```python
from build123d import *

# Parameters (mm, degrees)
SKETCH2_R           = 30
BOSS_EXTRUDE1_DEPTH = 30
SKETCH3_W           = 13.5
SKETCH3_H           = 15
CUT_EXTRUDE1_DEPTH  = 31
SKETCH4_W           = 33
SKETCH4_H           = 13.5
CUT_EXTRUDE2_DEPTH  = 10.5
SKETCH5_W           = 25
SKETCH5_H           = 13.5
CUT_EXTRUDE3_DEPTH  = 20.5
FILLET1_R           = 0.5
BOSS_EXTRUDE2_DEPTH = 2.5
SKETCH9_R           = 2.75
CUT_EXTRUDE4_DEPTH  = 3.5
SKETCH10_R          = 1.5
CUT_EXTRUDE5_DEPTH  = 5
FILLET2_R           = 2


with BuildPart() as part:
    # Sketch2 → Boss-Extrude1 (new body)
    with BuildSketch(Plane(origin=(0, 0, 0), x_dir=(1, 0, 0), z_dir=(0, 1, 0))):
        Circle(SKETCH2_R)
    extrude(amount=BOSS_EXTRUDE1_DEPTH)

    # Sketch3 → Cut-Extrude1 (cut, through all)
    with BuildSketch(Plane(origin=(0, 0, 0), x_dir=(0, 0, -1), z_dir=(1, 0, 0))):
        with Locations((0, 7.5)):
            Rectangle(SKETCH3_W, SKETCH3_H)
    extrude(amount=CUT_EXTRUDE1_DEPTH, mode=Mode.SUBTRACT)

    # Sketch4 → Cut-Extrude2 (cut)
    with BuildSketch(Plane(origin=(0, 30, 0), x_dir=(1, 0, 0), z_dir=(0, 1, 0))):
        with Locations((-5.5, 0)):
            Rectangle(SKETCH4_W, SKETCH4_H)
    extrude(amount=-CUT_EXTRUDE2_DEPTH, mode=Mode.SUBTRACT)

    # Sketch5 → Cut-Extrude3 (cut, through all)
    with BuildSketch(Plane(origin=(0, 19.5, 0), x_dir=(1, 0, 0), z_dir=(0, 1, 0))):
        with Locations((-5.5, 0)):
            Rectangle(SKETCH5_W, SKETCH5_H)
    extrude(amount=-CUT_EXTRUDE3_DEPTH, mode=Mode.SUBTRACT)

    # Sketch7 → Revolve1 (revolve)
    with BuildSketch(Plane.XY):
        with BuildLine():
            Line((30, 30), (28, 30))
            Line((28, 30), (28, 32))
            ThreePointArc((28, 32), (29, 33), (30, 32))
            Line((30, 32), (30, 30))
        make_face()
    revolve(axis=Axis((0, 34.959815409, 0), (0, -1, 0)))

    # Fillet1
    fillet1_edges = [part.edges().sort_by_distance(p)[0] for p in [
        (-28, 30, 0),
    ]]
    fillet(fillet1_edges, radius=FILLET1_R)

    # Sketch8 → Boss-Extrude2 (add)
    with BuildSketch(Plane(origin=(0, 0, 0), x_dir=(1, 0, 0), z_dir=(0, 1, 0))):
        with BuildLine():
            ThreePointArc((24.452034569, -17.380966757), (21.213203436, -21.213203436), (17.380966757, -24.452034569))
            Line((17.380966757, -24.452034569), (24.452034569, -31.523102381))
            ThreePointArc((24.452034569, -31.523102381), (31.523102381, -31.523102381), (31.523102381, -24.452034569))
            Line((31.523102381, -24.452034569), (24.452034569, -17.380966757))
        make_face()
        with BuildLine():
            ThreePointArc((-17.380966757, -24.452034569), (-21.213203436, -21.213203436), (-24.452034569, -17.380966757))
            Line((-24.452034569, -17.380966757), (-31.523102381, -24.452034569))
            ThreePointArc((-31.523102381, -24.452034569), (-31.523102381, -31.523102381), (-24.452034569, -31.523102381))
            Line((-24.452034569, -31.523102381), (-17.380966757, -24.452034569))
        make_face()
        with BuildLine():
            ThreePointArc((17.380966757, 24.452034569), (21.213203436, 21.213203436), (24.452034569, 17.380966757))
            Line((24.452034569, 17.380966757), (31.523102381, 24.452034569))
            ThreePointArc((31.523102381, 24.452034569), (31.523102381, 31.523102381), (24.452034569, 31.523102381))
            Line((24.452034569, 31.523102381), (17.380966757, 24.452034569))
        make_face()
        with BuildLine():
            ThreePointArc((-24.452034569, 17.380966757), (-21.213203436, 21.213203436), (-17.380966757, 24.452034569))
            Line((-17.380966757, 24.452034569), (-24.452034569, 31.523102381))
            ThreePointArc((-24.452034569, 31.523102381), (-31.523102381, 31.523102381), (-31.523102381, 24.452034569))
            Line((-31.523102381, 24.452034569), (-24.452034569, 17.380966757))
        make_face()
    extrude(amount=BOSS_EXTRUDE2_DEPTH)

    # Sketch9 → Cut-Extrude4 (cut, through all)
    with BuildSketch(Plane(origin=(0, 2.5, 0), x_dir=(1, 0, 0), z_dir=(0, 1, 0))):
        with Locations((-27.987568475, 27.987568475)):
            Circle(SKETCH9_R)
        with Locations((27.987568475, 27.987568475)):
            Circle(SKETCH9_R)
        with Locations((27.987568475, -27.987568475)):
            Circle(SKETCH9_R)
        with Locations((-27.987568475, -27.987568475)):
            Circle(SKETCH9_R)
    extrude(amount=-CUT_EXTRUDE4_DEPTH, mode=Mode.SUBTRACT)

    # Sketch10 → Cut-Extrude5 (cut)
    with BuildSketch(Plane(origin=(0, 19.5, 0), x_dir=(1, 0, 0), z_dir=(0, 1, 0))):
        with Locations((-20, 0)):
            Circle(SKETCH10_R)
        with Locations((9, 0)):
            Circle(SKETCH10_R)
    extrude(amount=-CUT_EXTRUDE5_DEPTH, mode=Mode.SUBTRACT)

    # Fillet2
    fillet2_edges = [part.edges().sort_by_distance(p)[0] for p in [
        (-21.213203436, 2.5, -21.213203436),
        (21.213203436, 2.5, 21.213203436),
        (-21.213203436, 2.5, 21.213203436),
        (21.213203436, 2.5, -21.213203436),
    ]]
    fillet(fillet2_edges, radius=FILLET2_R)


solid = part.part
```
Read the model definition and answer for the solid it produces. Units are mm, in the model's axes. A direction names the side the tool comes from. Give positions to 0.01 mm unless a question says otherwise; leave off trailing zeros. Loops run counter-clockwise (first coordinate to the right, second up) from the corner with the lowest first, then second, coordinate; pieces in that order, holes last.
Item 1: The part is cut by section B-B (y = 16.5). Write down the section's boundary in (x, z), and give its area (3 significant figures).
Item 2: The part is cut by section C-C (z = 0). Write down the section's boundary in (x, y).
Item 3: Each of these flat-tipped pins is pushed along its axis until it touches: pin 1 Ø10 at (x, y) = (-19, 25) entering from -Z; pin 2 Ø8 at (y, z) = (7.5, -24.5) entering from +X; pin 3 Ø4.5 at (x, z) = (-26.5, -25) entering from +Y; pin 4 Ø6 at (x, z) = (-22.5, 8.5) entering from -Y. Where does it stop, or does it pass through?
Item 4: For faces 4 (the flat face through (20.87, 1.22, 27.94)), 5 (the cylindrical face through (-21.5, 17.04, -0.07)), 6 (the flat face through (27.94, 1.22, -20.87)), 7 (the cylindrical face through (-30.014, 1.268, 26.129)), determine the directions among +Z, -Z, +X, -X, +Y, -Y from which every point of the face is accessible in a straight line to the end or side of a thin tool.
Item 5: The part is cut by section D-D (y = 23). Write down the section's boundary in (x, z).
Item 6: The mould has two halves that part along Z. Classify faces 1 (the flat face through (-26, 2.5, -24)), 2 (the flat face through (-20.87, 1.22, -27.94)), 3 (the flat face through (-18, 10, 0)): released by +Z, released by -Z, zero draft, split by the parting line, or undercut.
Item 7: The part is cut by section A-A (x = 0). Write down the section's boundary in (y, z), and give its area (3 significant figures).
Item 8: Find the intervals of material crossed by line 1 along Z through (x, y) = (0, 30.9); line 2 along Z through (x, y) = (27.5, 11.5); line 3 along X through (y, z) = (31, 5.5), in increasing order.
Taken from the geometry:
1. outline: circle Ø60 at (0, 0); hole circle Ø3 at (-20, 0); hole (-18, -6.75) - (7, -6.75) - (7, 6.75) - (-18, 6.75) - close; hole circle Ø3 at (9, 0)
1. area: 2,480 mm2
2. outline: (-30, 0) - (-18, 0) - (-18, 19.5) - (-18.5, 19.5) - (-18.5, 14.5) - (-21.5, 14.5) - (-21.5, 19.5) - (-22, 19.5) - (-22, 30) - (-27.5, 30) arc R0.5 cw to (-28, 30.5) - (-28, 32) arc R1 ccw to (-30, 32) - close; (7, 15) - (7.5, 15) - (7.5, 19.5) - (7, 19.5) - close; (10.5, 15) - (30, 15) - (30, 32) arc R1 ccw to (28, 32) - (28, 30.5) arc R0.5 cw to (27.5, 30) - (11, 30) - (11, 19.5) - (10.5, 19.5) - close
3. pin 1: stops at z = -26.53
3. pin 2: stops at x = 21.9
3. pin 3: stops at y = 2.5
3. pin 4: stops at y = 0
4. face 4: +Z, +Y, -Y
4. face 5: +Y
4. face 6: +X, +Y, -Y
4. face 7: +Y, -Y
5. outline: circle Ø60 at (0, 0); hole (-22, -6.75) - (11, -6.75) - (11, 6.75) - (-22, 6.75) - close
6. face 1: zero draft
6. face 2: released by -Z
6. face 3: undercut
7. outline: (0, -30) - (32, -30) arc R1 ccw to (32, -28) - (30.5, -28) arc R0.5 cw to (30, -27.5) - (30, -6.75) - (0, -6.75) - close; (0, 6.75) - (30, 6.75) - (30, 27.5) arc R0.5 cw to (30.5, 28) - (32, 28) arc R1 ccw to (32, 30) - (0, 30) - close
7. area: 1,410 mm2
8. line 1: z = -30 to -28, 28 to 30
8. line 2: z = -11.99 to -6.75, 6.75 to 11.99
8. line 3: x = -29.49 to -27.45, 27.45 to 29.49
